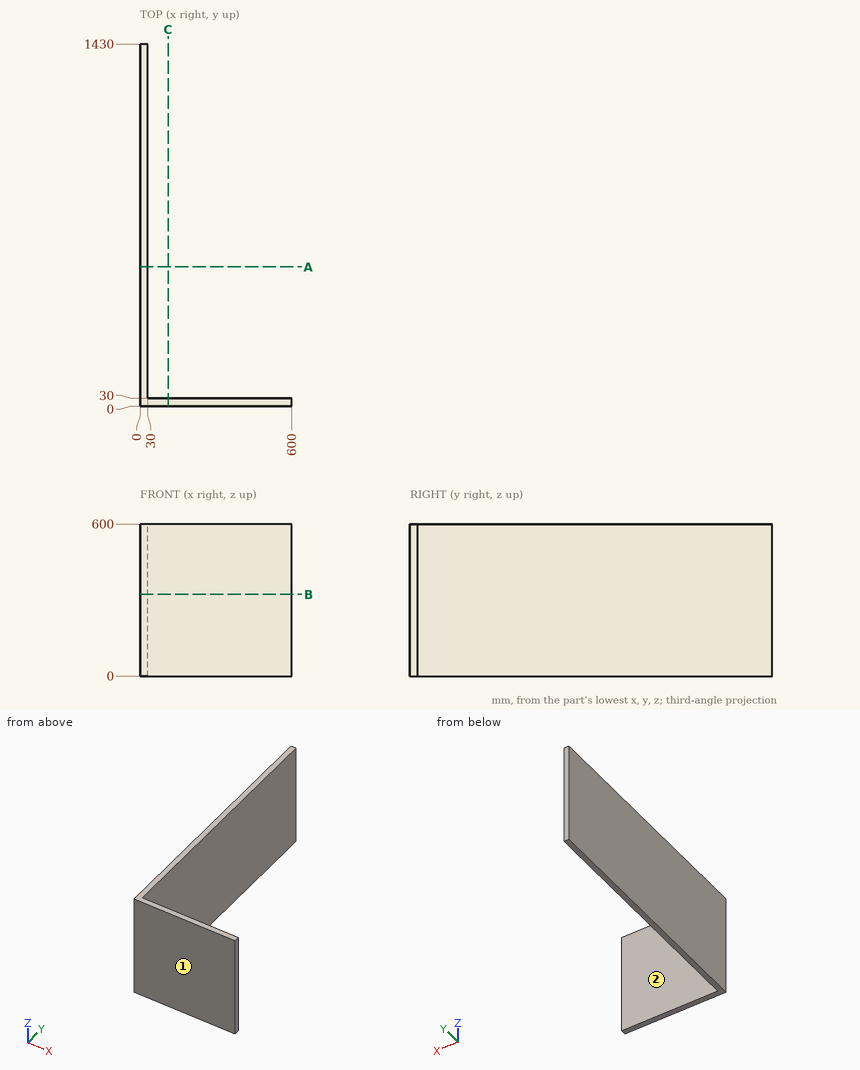
Job drawing, mm, ordinate dimensions from the low corner. One solid piece. A direction names the side the tool comes from. Round coordinates to 2 decimals unless told otherwise and drop trailing zeros. Write each loop counter-clockwise with the first axis right and the second up, starting at its lowest first coordinate (ties: lowest second). Pieces come first, ordered by that corner, then holes. Notation, with made-up numbers: M 4,73 L 25,73 A20 cw 25,103 Z; hole C -36,64.5 d7. An arc over 180 degrees is marked long. Return JSON: item names as keys, results as strings. Group by question number.
(1) Saw through at A-A on y = 550. Write the cut outline in (x, z), then the cut area to 3 significant figures.
(2) Saw through at B-B on z = 322.5. Write the cut outline in (x, y).
(3) Pin check, flat tips, straight feed: pin 1 Ø3 at (y, z) = (946.5, 338) entering from -X; pin 2 Ø1.5 at (x, z) = (468.5, 492) entering from +Y; pin 3 Ø4 at (y, z) = (197.5, 470.5) entering from +X. Stop position of each tip, or through.
(4) Drill centre line: probe 1 along Y at (x, z) = (373, 94). Where is it in solid material? Low to high.
(5) Which spindle directions (+Z, -Z, +X, -X, +Y, -Y) get a long thin tool onto all of the face, cutting with end or side? Do the marked faces 1 and 2. Say none if no direction does.
Returned:
{
 "1": {"outline": "M 0,0 L 30,0 L 30,600 L 0,600 Z", "area": "18,000 mm²"},
 "2": {"outline": "M 0,0 L 600,0 L 600,30 L 30,30 L 30,1430 L 0,1430 Z"},
 "3": {"pin 1": "x = 0", "pin 2": "y = 30", "pin 3": "x = 30"},
 "4": {"probe 1": "0 to 30"},
 "5": {"face 1": "+Z, -Z, +X, -X, -Y", "face 2": "+Z, -Z, +X, +Y"}
}
